Geometry check sheet. Reference: the model listing, model coordinates, mm. A direction names the side the tool comes from. Give positions to 0.01 mm unless a question says otherwise; leave off trailing zeros. Loops run counter-clockwise (first coordinate to the right, second up) from the corner with the lowest first, then second, coordinate; pieces in that order, holes last. Notation, with made-up numbers: (66.5, 19) -> (116.5, 19) arc R6 ccw to (116.5, 30) -> close; hole circle Ø11 at (1.5, 72.25). An arc over 180 degrees is marked (long way). Write item = value, one per line. Start each with the question number.
```python
from build123d import *

# Parameters (mm, degrees)
CUT_EXTRUDE1_DEPTH      = 201.445503114
CUT_EXTRUDE1_DEPTH_BACK = 201.445503114
SKETCH2_R               = 3.175


with BuildPart() as part:
    # Sketch1 → Revolve1 (revolve)
    with BuildSketch(Plane(origin=(0, 0, 0), x_dir=(0, 0, -1), z_dir=(1, 0, 0)), mode=Mode.PRIVATE) as revolve1_sk:
        with BuildLine():
            Line((-170.558103969, 61.982800726), (0, 25.4))
            Line((0, 25.4), (0, 20.6375))
            ThreePointArc((0, 20.6375), (14.592916197, 14.592916197), (20.6375, 0))
            Line((20.6375, 0), (19.05, 0))
            ThreePointArc((19.05, 0), (13.470384182, 13.470384182), (0, 19.05))
            Line((0, 19.05), (-12.7, 19.05))
            Line((-12.7, 19.05), (-12.7, 26.500401371))
            Line((-12.7, 26.500401371), (-177.8, 61.9125))
            Line((-177.8, 61.9125), (-177.8, 63.5))
            Line((-177.8, 63.5), (-176.773784801, 63.279888347))
            ThreePointArc((-176.773784801, 63.279888347), (-175.364378816, 63.379506676), (-174.226260414, 64.21678533))
            ThreePointArc((-174.226260414, 64.21678533), (-173.438552848, 64.958591119), (-172.456828691, 65.413538059))
            ThreePointArc((-172.456828691, 65.413538059), (-171.763807138, 65.28185552), (-171.45, 64.650076885))
            Line((-171.45, 64.650076885), (-171.45, 63.086283803))
            ThreePointArc((-171.45, 63.086283803), (-171.199147092, 62.376855612), (-170.558103969, 61.982800726))
        make_face()
    revolve(revolve1_sk.sketch.rotate(Axis((0, 0, 0), (0, 0, 1)), 90), axis=Axis((0, 0, 0), (0, 0, 1)))

    # Sketch2 → Cut-Extrude1 (cut, two sides: drawn at the far end of the back side and taken through both)
    with BuildSketch(Plane(origin=(0, 0, 0), x_dir=(1, 0, 0), z_dir=(0, 1, 0)).offset(-CUT_EXTRUDE1_DEPTH_BACK)):
        with Locations(Location((0, -95.25, 0), (0, 0, 124.156091497))):
            Circle(SKETCH2_R)
    extrude(amount=CUT_EXTRUDE1_DEPTH + CUT_EXTRUDE1_DEPTH_BACK, mode=Mode.SUBTRACT)


solid = part.part
```
1) Depth check by flat-ended pin: pin 1 Ø7.5 at (x, z) = (0, 95.25) entering from +Y; pin 2 Ø4 at (x, z) = (0, 95.25) entering from +Y; pin 3 Ø3 at (x, z) = (-2, 92.5) entering from -Y; pin 4 Ø3 at (x, y) = (-40.5, 51.5) entering from -Z. Enter the tip coordinate at first touch or a pass-through.
2) Tool access check on faces 1 (the cylindrical face through (1.67, -45.04, 97.95)), 2 (the cylindrical face through (4.13, 18.597, 6.439)), 3 (the flat face through (0, -21, 0)). Record the directions out of +Z, -Z, +X, -X, +Y, -Y that give a thin tool (end or side, any length) a straight path to the whole face; none if there is none.
3) Section check C-C (z = 119). Enter the section's corners in (x, y).
4) Thickness scan on line 1 (Y direction, x = -2, z = 76); line 2 (Y direction, x = 4, z = 125); line 3 (X direction, y = 12, z = 53.5). Record the ranges inside material, lowest first.
5) Section check B-B (z = 17). Enter the section's corners in (x, y).
6) Draft check along X on faces 4 (the conical face through (-20.043, 38.535, 84.085)), 5 (the flat face through (14, 61, 177.8)), 6 (the flat face through (11, 17, 12.7)). Enter one of: released by +X, released by -X, zero draft, split by the parting line, or undercut.
Check result:
q1.pin_1 = 46.63
q1.pin_2 = through
q1.pin_3 = -45.42
q1.pin_4 = 171.45
q2.face_1 = +Y, -Y
q2.face_2 = +Z
q2.face_3 = -Z
q3.outline = circle Ø101.85 at (0, 0); hole circle Ø98.6 at (0, 0)
q4.line_1 = -41.65 to -40.03, 40.03 to 41.65
q4.line_2 = -52.06 to -50.43, 50.43 to 52.06
q4.line_3 = -34.87 to -33.15, 33.15 to 34.87
q5.outline = circle Ø58.09 at (0, 0); hole circle Ø54.85 at (0, 0)
q6.face_4 = split by the parting line
q6.face_5 = zero draft
q6.face_6 = undercut
